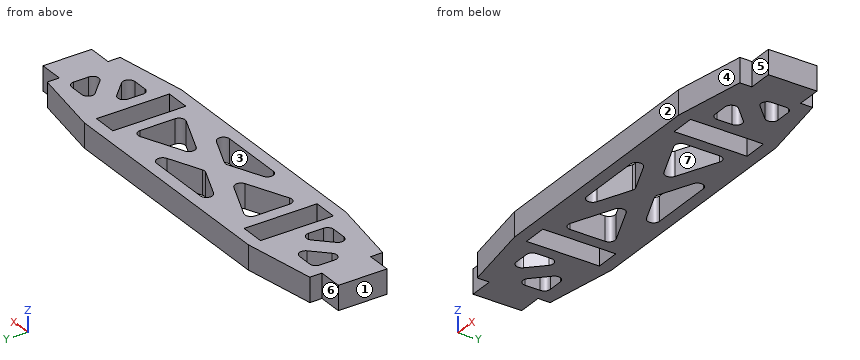
```python
from build123d import *

# Parameters (mm, degrees)
SKETCH1_W           = 6.35
SKETCH1_H           = 19.05
BOSS_EXTRUDE1_DEPTH = 3.175
CUT_EXTRUDE1_DEPTH  = 7.35
FILLET1_R           = 1.5875


with BuildPart() as part:
    # Sketch1 → Boss-Extrude1 (new body, symmetric)
    with BuildSketch(Plane.XY):
        Polygon((-50.8, -9.525), (-50.8, -6.35), (-57.15, -6.35), (-57.15, 6.35), (-50.8, 6.35), (-50.8, 9.525), (-31.75, 12.7), (31.75, 12.7), (50.8, 9.525), (50.8, 6.35), (57.15, 6.35), (57.15, -6.35), (50.8, -6.35), (50.8, -9.525), (31.75, -12.7), (-31.75, -12.7), align=None)
        with Locations((-28.575, 0)):
            Rectangle(SKETCH1_W, SKETCH1_H, mode=Mode.SUBTRACT)
        with Locations((28.575, 0)):
            Rectangle(SKETCH1_W, SKETCH1_H, mode=Mode.SUBTRACT)
    extrude(amount=BOSS_EXTRUDE1_DEPTH, both=True)

    # Sketch2 → Cut-Extrude1 (cut, through all)
    with BuildSketch(Plane.XY.offset(3.175)):
        Polygon((-38.292596045, 6.35), (-47.625, 6.35), (-47.625, -2.982403955), align=None)
        Polygon((-34.925, 2.982403955), (-44.257403955, -6.35), (-34.925, -6.35), align=None)
        Polygon((-22.225, -6.934277185), (-6.045019903, 0), (-22.225, 6.934277185), align=None)
        Polygon((-16.179980097, 9.525), (0, 2.590722815), (16.179980097, 9.525), align=None)
        Polygon((6.045019903, 0), (22.225, -6.934277185), (22.225, 6.934277185), align=None)
        Polygon((-16.179980097, -9.525), (16.179980097, -9.525), (0, -2.590722815), align=None)
        Polygon((44.257403955, -6.35), (34.925, 2.982403955), (34.925, -6.35), align=None)
        Polygon((47.625, 6.35), (38.292596045, 6.35), (47.625, -2.982403955), align=None)
    extrude(amount=-CUT_EXTRUDE1_DEPTH, mode=Mode.SUBTRACT)

    # Fillet1
    fillet1_edges = [part.edges().sort_by_distance(p)[0] for p in [
        (16.179980097, 9.525, 0),
        (0, 2.590722815, 0),
        (-16.179980097, 9.525, 0),
        (22.225, 6.934277185, 0),
        (22.225, -6.934277185, 0),
        (6.045019903, 0, 0),
        (-6.045019903, 0, 0),
        (-22.225, -6.934277185, 0),
        (-22.225, 6.934277185, 0),
        (-34.925, 2.982403955, 0),
        (-34.925, -6.35, 0),
        (-44.257403955, -6.35, 0),
        (38.292596045, 6.35, 0),
        (47.625, 6.35, 0),
        (47.625, -2.982403955, 0),
        (44.257403955, -6.35, 0),
        (34.925, -6.35, 0),
        (34.925, 2.982403955, 0),
        (0, -2.590722815, 0),
        (16.179980097, -9.525, 0),
        (-16.179980097, -9.525, 0),
        (-38.292596045, 6.35, 0),
        (-47.625, -2.982403955, 0),
        (-47.625, 6.35, 0),
    ]]
    fillet(fillet1_edges, radius=FILLET1_R)


solid = part.part
```
CAD build for the part. Positions are in the model's coordinates, mm. Face numbers are marked on the shaded views. A direction names the side the tool comes from. Coordinates: 2 decimals unless noted, no trailing zeros. Loops run counter-clockwise (first coordinate to the right, second up) from the corner with the lowest first, then second, coordinate; pieces in that order, holes last. Notation, with made-up numbers: (-7.5, 66) - (36.5, 66) arc R13 cw to (36.5, 72) - close; hole circle Ø10 at (31, 62). An arc over 180 degrees is marked (long way). Use CSV: the item, a comma, the result in double quotes. Start each with the question number.
Q1. 3-axis set-ups, long thin cutter, end or side, ignore diameter. For the marked faces 5, 6 and 7: which of +Z, -Z, +X, -X, +Y, -Y reach the whole face in a straight line?
Q2. Two-plate mould, pull along X, no slides. Class the marked faces 1, 2, 3 and 4: +X half, -X half, draft (parallel to the pull), parting line (faces both ways), or undercut.
Q3. Drop flat-ended pins along their axis: P1, Ø2, axis at y = -8, z = 0, coming from the +X side; P2, Ø1.2, axis at x = 43.5, z = 0, coming from the -Y side. Give the stop position or say it passes through.
Q4. Cut at A-A, the plane x = -14. List the corners of the cut face in (y, z) (3 decimals), then the cut area to 3 significant figures.
Q5. Cut at B-B, the plane z = 0.25. State how many separate pieces and enclosed holes the cut face has, then the cut area to 3 significant figures.
Q6. Probe probe 1 along Y at (x, z) = (8, -2) (3 decimals); probe 2 along Y at (x, z) = (20.5, -2.5); probe 3 along Y at (x, z) = (-30, -2.25) (3 decimals). List the from-to ranges inside material, lowest first. Write a range as from..to.
Here are the results:
1,face 5,"+Z, -Z, +X, -Y"
1,face 6,"+Z, -Z, -X, +Y"
1,face 7,"+Z, -Z"
2,face 1,"-X half"
2,face 2,"draft"
2,face 3,"undercut"
2,face 4,"+X half"
3,P1,"x = 50.8"
3,P2,"y = -10.84"
4,outline,"(-12.7, -3.175) - (-3.409, -3.175) - (-3.409, 3.175) - (-12.7, 3.175) - close; (3.409, -3.175) - (12.7, -3.175) - (12.7, 3.175) - (3.409, 3.175) - close"
4,area,"118 mm2"
5,separate pieces,"1"
5,enclosed holes,"10"
5,area,"1,830 mm2"
6,probe 1,"-12.7..-9.525, -6.019..6.019, 9.525..12.7"
6,probe 2,"-12.7..-6.11, 6.11..12.7"
6,probe 3,"-12.7..-9.525, 9.525..12.7"
